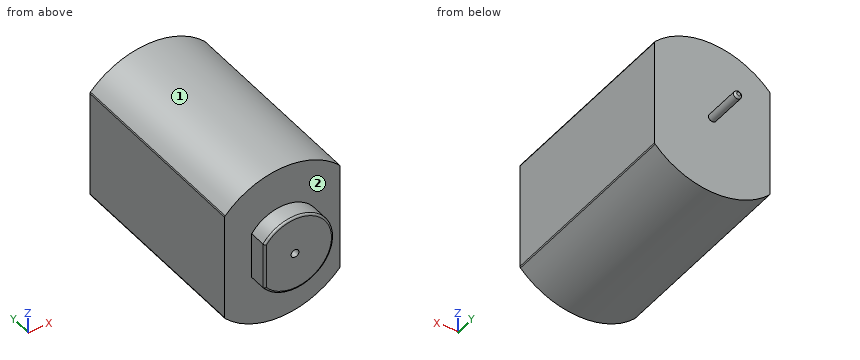
from build123d import *

# Parameters (mm, degrees)
F1_DEPTH = 24.87
F0_R     = 0.5
F2_DEPTH = 27.2
F3_DEPTH = 4.85
F4_R     = 0.254


with BuildPart() as f1:
    # F0 (on Front) → F1 (new body)
    with BuildSketch(Plane.XZ):
        with BuildLine():
            Line((-7.4, 6.95), (-7.4, -6.95))
            ThreePointArc((-7.4, -6.95), (0, -10.1519702521), (7.4, -6.95))
            Line((7.4, -6.95), (7.4, 6.95))
            ThreePointArc((7.4, 6.95), (0, 10.1519702521), (-7.4, 6.95))
        make_face()
        with BuildLine():
            ThreePointArc((-3.935, 2.9782545224), (4.935, 0), (-3.935, -2.9782545224))
            Line((-3.935, -2.9782545224), (-3.935, 2.9782545224))
        make_face(mode=Mode.SUBTRACT)
    extrude(amount=F1_DEPTH)

    # F0 (on Front) → F2 (join)
    with BuildSketch(Plane.XZ):
        with BuildLine():
            Line((-3.935, 2.9782545224), (-3.935, -2.9782545224))
            ThreePointArc((-3.935, -2.9782545224), (4.935, 0), (-3.935, 2.9782545224))
        make_face()
        Circle(F0_R, mode=Mode.SUBTRACT)
    extrude(amount=F2_DEPTH)

    # F0 (on Front) → F3 (join, symmetric)
    with BuildSketch(Plane.XZ):
        Circle(F0_R)
    extrude(amount=F3_DEPTH, both=True)

    # F4
    f4_edges = [f1.edges().sort_by_distance(p)[0] for p in [
        (-3.935, -27.2, 0),
        (4.935, -27.2, 0),
        (7.4, -12.435, -6.95),
        (7.4, -12.435, 6.95),
        (-7.4, -12.435, 6.95),
        (-7.4, -12.435, -6.95),
        (-0.5, 4.85, 0),
    ]]
    fillet(f4_edges, radius=F4_R)


solid = f1.part
CAD build for the part. Positions are in the model's coordinates, mm. Face numbers are marked on the shaded views. A direction names the side the tool comes from. Round coordinates to 2 decimals unless told otherwise and drop trailing zeros. Loops run counter-clockwise (first coordinate to the right, second up) from the corner with the lowest first, then second, coordinate; pieces in that order, holes last. Notation, with made-up numbers: M -14,16.25 L 38,16.25 A12 cw 38,29.25 Z; hole C 67,28.25 d7. An arc over 180 degrees is marked long. One line per question, with ' | ' between items. Start each with the question number.
Item 1: Cut at B-B, the plane y = -1. Write the cut outline in (x, z), plus the area to 3 significant figures.
Item 2: Cut at C-C, the plane x = -5.75. Write the cut outline in (y, z), plus the area to 3 significant figures.
Item 3: Which spindle directions (+Z, -Z, +X, -X, +Y, -Y) get a long thin tool onto all of the face, cutting with end or side? Do the marked faces 1 and 2. Say none if no direction does.
Item 4: Cut at A-A, the plane y = -10.5. Write the cut outline in (x, z).
Item 5: Wall check: line 1 (Y direction, x = 5.75, z = -2.5); line 2 (Y direction, x = 4.25, z = -0.25); line 3 (X direction, y = -4.5, z = -7.5). Give the ranges that are in metal, low to high.
Item 6: Cut at D-D, the plane z = -8.25. Write the cut outline in (x, y), plus the area to 3 significant figures.
Item 7: Pin check, flat tips, straight feed: pin 1 Ø2 at (x, z) = (-3.5, 5) entering from -Y; pin 2 Ø0.5 at (x, z) = (0, 0) entering from -Y; pin 3 Ø1 at (y, z) = (-25.5, 0) entering from -X (3 decimals). Stop position of each tip, or through.
Responses:
1) outline: M -7.4,-6.85 A0.25 ccw -7.33,-7.02 A10.15 ccw 7.33,-7.02 A0.25 ccw 7.4,-6.85 L 7.4,6.85 A0.25 ccw 7.33,7.02 A10.15 ccw -7.33,7.02 A0.25 ccw -7.4,6.85 Z | area: 271 mm²
2) outline: M -24.87,-8.37 L 0,-8.37 L 0,8.37 L -24.87,8.37 Z | area: 416 mm²
3) face 1: +Z, +Y, -Y | face 2: -Y
4) outline: M -7.4,-6.85 A0.25 ccw -7.33,-7.02 A10.15 ccw 7.33,-7.02 A0.25 ccw 7.4,-6.85 L 7.4,6.85 A0.25 ccw 7.33,7.02 A10.15 ccw -7.33,7.02 A0.25 ccw -7.4,6.85 Z; hole C 0,0 d1
5) line 1: y = -24.87 to 0 | line 2: y = -27.2 to 0 | line 3: x = -6.84 to 6.84
6) outline: M -5.92,-24.87 L 5.92,-24.87 L 5.92,0 L -5.92,0 Z | area: 294 mm²
7) pin 1: stops at y = -24.87 | pin 2: stops at y = -4.85 | pin 3: stops at x = -3.935
